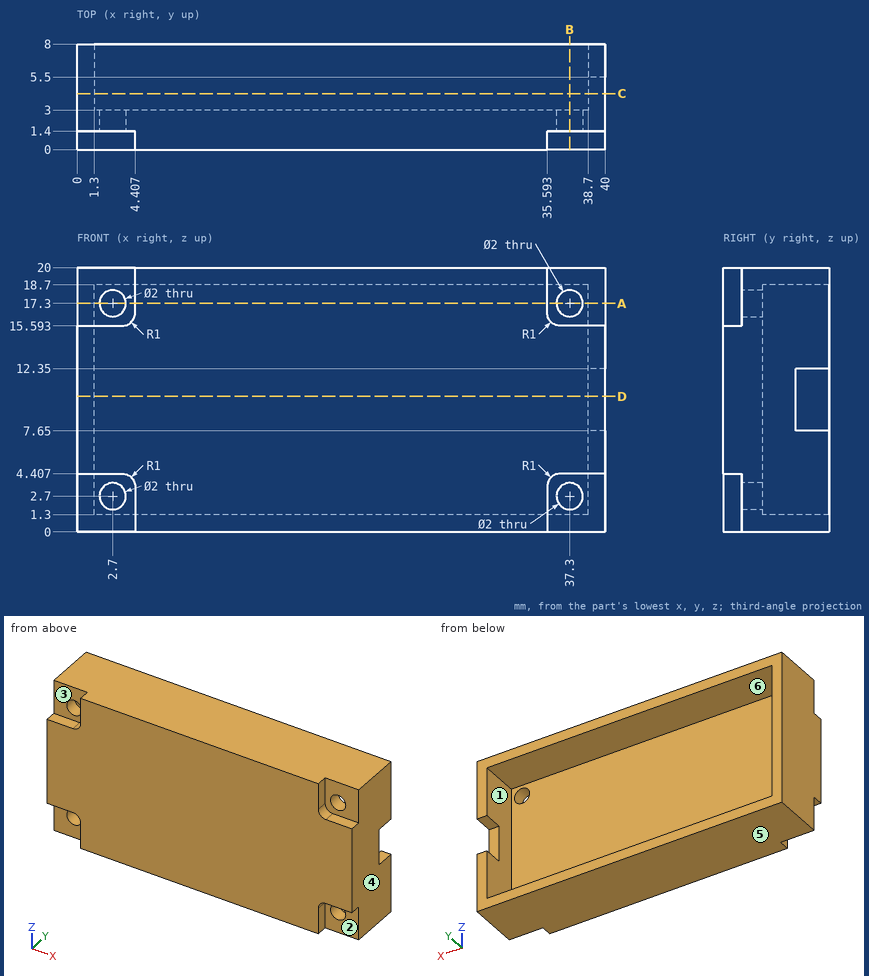
Source: three-view drawing plus pictorial views. Frame: mm from the lowest corner of the part. A direction names the side the tool comes from. Coordinates: 2 decimals unless noted, no trailing zeros. Order: outer loops, then holes, each group sorted by start corner. A loop starts at its lowest first (then second) coordinate and runs counter-clockwise, first axis right, second up. Notation, with made-up numbers: M 49,79.5 L 97,79.5 A22 ccw 97,88.5 Z; hole C -39.75,74 d7. An arc over 180 degrees is marked long. Answer in a Markdown table with one row per item.
(1) Material intervals for line 1 (X direction, y = 2, z = 2.75); line 2 (X direction, y = 4.75, z = 8.5); line 3 (Z direction, x = 4, y = 5), sorted ascending. Write a range as [from, to].
Numbers:
| item | result |
|---|---|
| line 1 | x = [0, 1.7], [3.7, 36.3], [38.3, 40] |
| line 2 | x = [0, 1.3], [38.7, 40] |
| line 3 | z = [0, 1.3], [18.7, 20] |
(2) Contact query for flat-ended pins moving along their axis: pin 1 Ø0.7 at (x, y) = (1, 1) entering from -Z; pin 2 Ø1.4 at (x, z) = (39.5, 9) entering from +Y; pin 3 Ø4 at (x, y) = (23, 4) entering from -Z; pin 4 Ø1.1 at (y, z) = (0.5, 18) entering from -X. Output: stop coordinate, or through.
Numbers:
| item | result |
|---|---|
| pin 1 | stops at z = 4.41 |
| pin 2 | stops at y = 5.5 |
| pin 3 | stops at z = 0 |
| pin 4 | stops at x = 4.41 |
(3) Section query D-D, the plane z = 10.25. Output: boundary loops of the cut face in (x, y).
Numbers:
| item | result |
|---|---|
| outline | M 0,0 L 40,0 L 40,5.5 L 38.7,5.5 L 38.7,3 L 1.3,3 L 1.3,8 L 0,8 Z |
(4) Access query for the marked faces 1, 2 and 3. Directions: +Z, -Z, +X, -X, +Y, -Y. A direction counts if a zero-diameter tool reaches every point of the face in a straight line with its end or side. Return the directions, or none.
Numbers:
| item | result |
|---|---|
| face 1 | +Y |
| face 2 | -Z, +X, -Y |
| face 3 | +Z, -X, -Y |
(5) Section query A-A, the plane z = 17.3. Output: boundary loops of the cut face in (x, y), plus the area to 3 significant figures.
Numbers:
| item | result |
|---|---|
| outline | M 0,1.4 L 1.7,1.4 L 1.7,3 L 1.3,3 L 1.3,8 L 0,8 Z; M 3.7,1.4 L 4.41,1.4 L 4.41,0 L 35.59,0 L 35.59,1.4 L 36.3,1.4 L 36.3,3 L 3.7,3 Z; M 38.3,1.4 L 40,1.4 L 40,8 L 38.7,8 L 38.7,3 L 38.3,3 Z |
| area | 114 mm^2 |
(6) Section query C-C, the plane y = 4.25. Output: boundary loops of the cut face in (x, z).
Numbers:
| item | result |
|---|---|
| outline | M 0,0 L 40,0 L 40,20 L 0,20 Z; hole M 1.3,1.3 L 38.7,1.3 L 38.7,18.7 L 1.3,18.7 Z |
(7) Section query B-B, the plane x = 37.3. Output: boundary loops of the cut face in (y, z).
Numbers:
| item | result |
|---|---|
| outline | M 0,4.41 L 1.4,4.41 L 1.4,3.7 L 3,3.7 L 3,16.3 L 1.4,16.3 L 1.4,15.59 L 0,15.59 Z; M 1.4,0 L 8,0 L 8,1.3 L 3,1.3 L 3,1.7 L 1.4,1.7 Z; M 1.4,18.3 L 3,18.3 L 3,18.7 L 8,18.7 L 8,20 L 1.4,20 Z |
(8) Draft query along X for the marked faces 4, 5 and 6. Return one class per face: pulls with the +X half, pulls with the -X half, needs draft (parallel to the pull), parting line crosses it, or undercut.
Numbers:
| item | result |
|---|---|
| face 4 | pulls with the +X half |
| face 5 | needs draft |
| face 6 | undercut |
